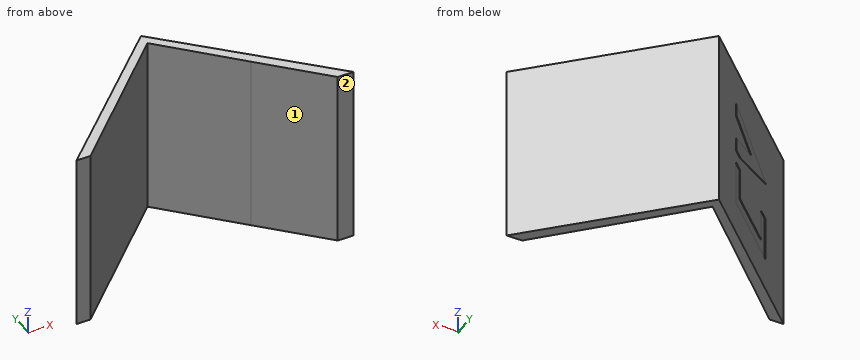
Autodesk Inventor part; units mm, degrees
ref_plane "Plano de trabajo1" through (0, 215, -283.5) normal (0.7021908, -0.7119888, 0) x (0, 0, 1)
ref_plane "YZ Plane" through (0, 0, 0) normal (1, 0, 0) x (0, 1, 0)
ref_plane "XZ Plane" through (0, 0, 0) normal (0, 1, 0) x (-1, 0, 0)
sketch "Boceto2" plane through (0, 0, 0) normal (0, 0, 1) x (1, 0, 0)
  line L0 (0, 0) -> (196, 0)
  line L1 (0, 0) -> (-196, 0)
  line L2 (0, 0) -> (0, 215)
  line L3 (-196, 0) -> (-218, 0)
  line L4 (-218, 0) -> (0, 215)
  line L5 (-263.5923, -44.9649) -> (-252.2786, -56.2786)
  line L6 (-263.5923, -44.9649) -> (-247.5923, -44.9649) construction
  line L7 (-252.2786, -56.2786) -> (0, 196)
  line L8 (-252.2786, -56.2786) -> (-196, 0)
  line L9 (196, 0) -> (221, 0)
  line L10 (221, 0) -> (0, 215)
  line L11 (117.9791, 100.2239) -> (106.6654, 88.9102)
  line L12 (117.9791, 100.2239) -> (133.9791, 100.2239) construction
  line L13 (106.6654, 88.9102) -> (0, 196)
  line L14 (106.6654, 88.9102) -> (196, 0)
  dimension "d0" = 196
  dimension "d1" = 196
  dimension "d2" = 215
  dimension "d3" = 22
  dimension "d4" = 16
  dimension "d5" = 45
  dimension "d6" = 25
  dimension "d7" = 16
  dimension "d8" = 135
extrude "Extrusión1" add sketch "Boceto2" against normal blind 283.5 contours L14 L11 L10 L9 | L3 L4 L2 L7 | L2 L10 L11 L13
ref_plane "Plano de trabajo1" through (0, 215, -283.5) normal (0.7021908, -0.7119888, 0) x (0, 0, 1)
sketch "Boceto3" plane through (0, 215, -283.5) normal (0.7021908, -0.7119888, 0) x (0, 0, 1)
  line L0 (283.5, 150.971) -> (0, 150.971)
  line L1 (0, 306.1846) -> (0, 0)
  line L2 (283.5, -6.3785) -> (0, -6.3785)
  line L3 (141.75, 150.971) -> (141.75, 0)
  line L4 (283.5, 0) -> (0, 0)
  line L5 (141.75, 0) -> (141.75, 80)
  line L6 (121.75, 80) -> (51.75, 80)
  line L7 (51.75, 80) -> (51.75, 220)
  line L8 (51.75, 220) -> (121.75, 220)
  line L9 (121.75, 200) -> (71.75, 200)
  line L10 (71.75, 200) -> (71.75, 100)
  line L11 (71.75, 100) -> (121.75, 100)
  line L12 (141.75, 80) -> (161.75, 80)
  line L13 (181.75, 220) -> (141.75, 100)
  line L14 (221.75, 80) -> (181.75, 220)
  line L15 (221.75, 80) -> (201.75, 80)
  line L16 (201.75, 80) -> (181.75, 150.971)
  line L17 (161.75, 80) -> (181.75, 150.971)
  line L18 (141.75, 80) -> (135.0833, 80)
  line L19 (121.75, 80) -> (121.75, 220)
  line L20 (135.0833, 80) -> (142.2633, 101.5399)
  point P0 (141.75, 220)
  point P1 (141.75, 200)
  dimension "d28" = 90
  dimension "d29" = 100
  dimension "d30" = 70
  dimension "d31" = 20
extrude "Extrusión2" cut sketch "Boceto3" along normal blind 1 contours L10 L11 L19 L6 L7 L0 | L0 L7 L8 L19 L9 L10
extrude "Extrusión3" add sketch "Boceto3" against normal blind 1 contours L14 L15 L16 L0 | L0 L13 L14 | L17 L12 L3 L13 L0
properties part number "TABLERO"
The listing builds one solid part. Answer for the finished solid, in the listing's coordinates (mm). Face numbers are marked on the shaded views. A direction names the side the tool comes from. Coordinates: 2 decimals unless noted, no trailing zeros. Write each loop counter-clockwise with the first axis right and the second up, starting at its lowest first coordinate (ties: lowest second). Pieces come first, ordered by that corner, then holes. Notation, with made-up numbers: (58, 81) - (114, 81) arc R12 ccw to (114, 91) - close; hole circle Ø2 at (38, 62). An arc over 180 degrees is marked (long way). Answer as CSV lines item,"result".
1. A tool of negligible diameter and unlimited length cuts with its end or side. For the marked faces 1 and 2, from which of +Z, -Z, +X, -X, +Y, -Y can it reach the whole face along a straight path? Write none if from no direction.
Computed values:
face 1,"+Z, -Z, -Y"
face 2,"+Z, -Z, +X, -X, -Y"
2. Find section D-D (y = 26). Give the vertices of the cut face in (x, z), plus the area to 3 significant figures.
Computed values:
outline,"(-191.64, -283.5) - (-170, -283.5) - (-170, 0) - (-191.64, 0) - close; (169.88, -283.5) - (194.27, -283.5) - (194.27, 0) - (169.88, 0) - close"
area,"13,100 mm²"
3. Find section C-C (x = -148). Give the vertices of the cut face in (y, z).
Computed values:
outline,"(48, -283.5) - (69.04, -283.5) - (69.04, -231.75) - (67.63, -231.75) - (67.63, -161.75) - (69.04, -161.75) - (69.04, -105.79) - (70.44, -106.12) - (70.44, -98) - (69.04, -98.28) - (69.04, 0) - (48, 0) - close"
4. Given P1, Ø5, axis at x = -15, z = -125, coming from the -Y side; P2, Ø2, axis at y = 146.5, z = -152, coming from the -X side; P3, Ø2, axis at y = 104, z = -48, coming from the -X side, each flat-ended and moving along its own axis, determine where each tip first touches the part or whether it passes through.
Computed values:
P1,"stops at y = 178.5"
P2,"stops at x = -70.47"
P3,"stops at x = -113.56"
5. Find section B-B (z = -262). Give the vertices of the cut face in (x, y), plus the area to 3 significant figures.
Computed values:
outline,"(-218, 0) - (-196, 0) - (0, 196) - (106.67, 88.91) - (196, 0) - (221, 0) - (0, 215) - close"
area,"8,820 mm²"
6. Find section A-A (y = 185). Give the vertices of the cut face in (x, z).
Computed values:
outline,"(-30.42, -283.5) - (-11, -283.5) - (-11, 0) - (-30.42, 0) - close; (10.96, -283.5) - (30.84, -283.5) - (30.84, 0) - (10.96, 0) - close"
7. Straight lines are drawn through the part: line 1 (X direction, y = 109, z = -134); line 2 (X direction, y = 96, z = -41); line 3 (Y direction, x = 84.5, z = -218). For each, find the intervals that lie inside material, in ascending order. Write a range as [from, to].
Computed values:
line 1,"x = [-107.48, -87], [86.66, 108.96]"
line 2,"x = [-120.66, -100], [99.6, 122.32]"
line 3,"y = [111.16, 132.79]"
